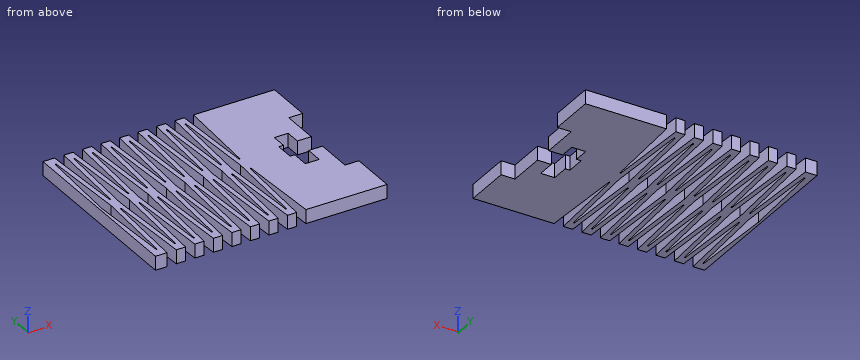
from build123d import *

# Parameters (mm, degrees)
EXTRUDE_1_DEPTH = 1.5


with BuildPart() as part:
    # 草图1 → 凸台-拉伸1 (new body, symmetric)
    with BuildSketch(Plane.XY):
        with BuildLine():
            Line((-22.5, 20), (-25, 20))
            Line((-25, 20), (-25, -20))
            Line((-25, -20), (-22.5, -20))
            Line((-22.5, -20), (-21.599875234, -1.997504678))
            ThreePointArc((-21.599875234, -1.997504678), (-21.5, -1.902498439), (-21.400124766, -1.997504678))
            Line((-21.400124766, -1.997504678), (-20.5, -20))
            Line((-20.5, -20), (-18.5, -20))
            Line((-18.5, -20), (-17.599875234, -1.997504678))
            ThreePointArc((-17.599875234, -1.997504678), (-17.5, -1.902498439), (-17.400124766, -1.997504678))
            Line((-17.400124766, -1.997504678), (-16.5, -20))
            Line((-16.5, -20), (-14.5, -20))
            Line((-14.5, -20), (-13.599875234, -1.997504678))
            ThreePointArc((-13.599875234, -1.997504678), (-13.5, -1.902498439), (-13.400124766, -1.997504678))
            Line((-13.400124766, -1.997504678), (-12.5, -20))
            Line((-12.5, -20), (-10.5, -20))
            Line((-10.5, -20), (-9.599875234, -1.997504678))
            ThreePointArc((-9.599875234, -1.997504678), (-9.5, -1.902498439), (-9.400124766, -1.997504678))
            Line((-9.400124766, -1.997504678), (-8.5, -20))
            Line((-8.5, -20), (-6.5, -20))
            Line((-6.5, -20), (-5.599875234, -1.997504678))
            ThreePointArc((-5.599875234, -1.997504678), (-5.5, -1.902498439), (-5.400124766, -1.997504678))
            Line((-5.400124766, -1.997504678), (-4.5, -20))
            Line((-4.5, -20), (-2.5, -20))
            Line((-2.5, -20), (-1.599875234, -1.997504678))
            ThreePointArc((-1.599875234, -1.997504678), (-1.5, -1.902498439), (-1.400124766, -1.997504678))
            Line((-1.400124766, -1.997504678), (-0.5, -20))
            Line((-0.5, -20), (1.5, -20))
            Line((1.5, -20), (2.400124766, -1.997504678))
            ThreePointArc((2.400124766, -1.997504678), (2.5, -1.902498439), (2.599875234, -1.997504678))
            Line((2.599875234, -1.997504678), (3.5, -20))
            Line((3.5, -20), (5.5, -20))
            Line((5.5, -20), (6.400124766, -1.997504678))
            ThreePointArc((6.400124766, -1.997504678), (6.5, -1.902498439), (6.599875234, -1.997504678))
            Line((6.599875234, -1.997504678), (7.5, -20))
            Line((7.5, -20), (25, -20))
            Line((25, -20), (25, -10))
            Line((25, -10), (22, -10))
            Line((22, -10), (22, -2))
            Line((22, -2), (19, -2))
            Line((19, -2), (19, -5.769694942))
            Line((19, -5.769694942), (16, -5.769694942))
            Line((16, -5.769694942), (16, -2))
            Line((16, -2), (15, -2))
            Line((15, -2), (15, 2))
            Line((15, 2), (16, 2))
            Line((16, 2), (16, 5.265909841))
            Line((16, 5.265909841), (19, 5.265909841))
            Line((19, 5.265909841), (19, 2))
            Line((19, 2), (22, 2))
            Line((22, 2), (22, 10))
            Line((22, 10), (25, 10))
            Line((25, 10), (25, 20))
            Line((25, 20), (7.5, 20))
            Line((7.5, 20), (6.599875234, 1.997504678))
            ThreePointArc((6.599875234, 1.997504678), (6.5, 1.902498439), (6.400124766, 1.997504678))
            Line((6.400124766, 1.997504678), (5.5, 20))
            Line((5.5, 20), (3.5, 20))
            Line((3.5, 20), (2.599875234, 1.997504678))
            ThreePointArc((2.599875234, 1.997504678), (2.5, 1.902498439), (2.400124766, 1.997504678))
            Line((2.400124766, 1.997504678), (1.5, 20))
            Line((1.5, 20), (-0.5, 20))
            Line((-0.5, 20), (-1.400124766, 1.997504678))
            ThreePointArc((-1.400124766, 1.997504678), (-1.5, 1.902498439), (-1.599875234, 1.997504678))
            Line((-1.599875234, 1.997504678), (-2.5, 20))
            Line((-2.5, 20), (-4.5, 20))
            Line((-4.5, 20), (-5.400124766, 1.997504678))
            ThreePointArc((-5.400124766, 1.997504678), (-5.5, 1.902498439), (-5.599875234, 1.997504678))
            Line((-5.599875234, 1.997504678), (-6.5, 20))
            Line((-6.5, 20), (-8.5, 20))
            Line((-8.5, 20), (-9.400124766, 1.997504678))
            ThreePointArc((-9.400124766, 1.997504678), (-9.5, 1.902498439), (-9.599875234, 1.997504678))
            Line((-9.599875234, 1.997504678), (-10.5, 20))
            Line((-10.5, 20), (-12.5, 20))
            Line((-12.5, 20), (-13.400124766, 1.997504678))
            ThreePointArc((-13.400124766, 1.997504678), (-13.5, 1.902498439), (-13.599875234, 1.997504678))
            Line((-13.599875234, 1.997504678), (-14.5, 20))
            Line((-14.5, 20), (-16.5, 20))
            Line((-16.5, 20), (-17.400124766, 1.997504678))
            ThreePointArc((-17.400124766, 1.997504678), (-17.5, 1.902498439), (-17.599875234, 1.997504678))
            Line((-17.599875234, 1.997504678), (-18.5, 20))
            Line((-18.5, 20), (-20.5, 20))
            Line((-20.5, 20), (-21.400124766, 1.997504678))
            ThreePointArc((-21.400124766, 1.997504678), (-21.5, 1.902498439), (-21.599875234, 1.997504678))
            Line((-21.599875234, 1.997504678), (-22.5, 20))
        make_face()
        Polygon((4.599875234, 18.002495322), (5.5, 0), (4.599875234, -18.002495322), (4.400124766, -18.002495322), (3.5, 0), (4.400124766, 18.002495322), align=None, mode=Mode.SUBTRACT)
        Polygon((0.599875234, -18.002495322), (0.400124766, -18.002495322), (-0.5, 0), (0.400124766, 18.002495322), (0.599875234, 18.002495322), (1.5, 0), align=None, mode=Mode.SUBTRACT)
        Polygon((-3.400124766, -18.002495322), (-3.599875234, -18.002495322), (-4.5, 0), (-3.599875234, 18.002495322), (-3.400124766, 18.002495322), (-2.5, 0), align=None, mode=Mode.SUBTRACT)
        Polygon((-7.400124766, -18.002495322), (-7.599875234, -18.002495322), (-8.5, 0), (-7.599875234, 18.002495322), (-7.400124766, 18.002495322), (-6.5, 0), align=None, mode=Mode.SUBTRACT)
        Polygon((-11.400124766, -18.002495322), (-11.599875234, -18.002495322), (-12.5, 0), (-11.599875234, 18.002495322), (-11.400124766, 18.002495322), (-10.5, 0), align=None, mode=Mode.SUBTRACT)
        Polygon((-15.400124766, -18.002495322), (-15.599875234, -18.002495322), (-16.5, 0), (-15.599875234, 18.002495322), (-15.400124766, 18.002495322), (-14.5, 0), align=None, mode=Mode.SUBTRACT)
        Polygon((-19.400124766, -18.002495322), (-19.599875234, -18.002495322), (-20.5, 0), (-19.599875234, 18.002495322), (-19.400124766, 18.002495322), (-18.5, 0), align=None, mode=Mode.SUBTRACT)
        Polygon((-23.400124766, -18.002495322), (-23.599875234, -18.002495322), (-24.5, 0), (-23.599875234, 18.002495322), (-23.400124766, 18.002495322), (-22.5, 0), align=None, mode=Mode.SUBTRACT)
    extrude(amount=EXTRUDE_1_DEPTH, both=True)


solid = part.part
Geometry: final body of the model. Coordinates: model frame, mm. Give positions to 0.01 mm unless a question says otherwise; leave off trailing zeros. Answer in a Markdown table with one row per item. Add a question column.
(1) Section A-A on y = 4. State how many separate pieces and enclosed holes the cut face has, and give its area (3 significant figures).
(2) Ray query, line 1 (Y direction, x = 20, z = 0.8); line 2 (Y direction, x = 23, z = 1); line 3 (Y direction, x = -9.5, z = -1.3). Return the intervals inside material, ascending.
(3) First-contact query: pin 1 (1.5 mm diameter, centred on y = -7, z = -0.5, fed in from +X). Flat tip, straight axial feed; report the tip coordinate or a pass-through.
Result set:
| question | item | result |
|---|---|---|
| 1 | separate pieces | 18 |
| 1 | enclosed holes | 0 |
| 1 | area | 84.0 mm^2 |
| 2 | line 1 | y = -20 to -2, 2 to 20 |
| 2 | line 2 | y = -20 to -10, 10 to 20 |
| 2 | line 3 | y = -1.9 to 1.9 |
| 3 | pin 1 | stops at x = 22 |
